Autodesk Fusion 360 part; units mm, degrees
sketch "Sketch1" plane through (0, 0, 0) normal (1, 0, 0) x (0, 0, -1)
  line L0 (0, 0) -> (-18.75, 0)
  line L1 (-18.75, 0) -> (-18.75, 20.75)
  line L2 (-18.75, 20.75) -> (0, 20.75)
  line L3 (0, 20.75) -> (0, 0)
  line L4 (-18.75, 20.75) -> (-18.75, 19)
  line L5 (-18.75, 0) -> (-18.75, 1.4)
  line L6 (-18.75, 19) -> (-22.75, 19)
  line L7 (-22.75, 19) -> (-22.75, 1.4)
  line L8 (-22.75, 1.4) -> (-18.75, 1.4)
  line L9 (-18.75, 1.4) -> (-18.75, 19)
  line L10 (-22.75, 19) -> (-22.75, 23.35)
  line L11 (-22.75, 1.4) -> (-22.75, -3.85)
  line L12 (-22.75, 23.35) -> (-60.15, 23.35)
  line L13 (-60.15, 23.35) -> (-60.15, -3.85)
  line L14 (-60.15, -3.85) -> (-22.75, -3.85)
  line L15 (-22.75, -3.85) -> (-22.75, 23.35)
  dimension "d1" = 18.75
  dimension "d2" = 20.75
  dimension "d4" = 1.75
  dimension "d6" = 4
  dimension "d7" = 4.35
  dimension "d9" = 37.4
sketch "Sketch3" plane through (0, 0, 0) normal (1, 0, 0) x (0, 0, -1)
  line L0 (-60.15, -3.85) -> (-60.15, 7.15)
  line L1 (-60.15, 7.15) -> (-39.15, 7.15)
  line L2 (-60.15, -3.85) -> (-22.75, -3.85)
  line L3 (-39.15, 7.15) -> (-39.15, -3.85)
  point P0 (-60.15, -3.85)
  dimension "d10" = 11
  dimension "d11" = 21
extrude "Extrude1" add sketch "Sketch3" along normal blind 6.15 makes body 1
sketch "Sketch4" plane through (6.15, 0, 0) normal (1, 0, 0) x (0, 0, -1)
  line L0 (-60.15, -3.85) -> (-39.15, -3.85)
  line L1 (-39.15, -3.85) -> (-39.15, 7.15)
  line L2 (-39.15, 7.15) -> (-60.15, 7.15)
  line L3 (-60.15, 7.15) -> (-60.15, -3.85)
  line L4 (-60.15, -3.85) -> (-18.75, -3.85)
  line L5 (-18.75, -3.85) -> (-18.75, 7.15)
  line L6 (-18.75, 7.15) -> (-60.15, 7.15)
  line L7 (-60.15, 7.15) -> (-60.15, -3.85)
  line L8 (-18.75, 1.4) -> (-18.75, 19)
extrude "Extrude2" add sketch "Sketch4" along normal blind 1.6 bodies 1
sketch "Sketch5" plane through (7.75, 0, 0) normal (1, 0, 0) x (0, 0, -1)
  line L0 (-18.75, -3.85) -> (-18.75, 7.15)
  line L1 (-18.75, 7.15) -> (-60.15, 7.15)
  line L2 (-60.15, 7.15) -> (-60.15, -3.85)
  line L3 (-60.15, -3.85) -> (-18.75, -3.85)
  line L4 (-60.15, -3.85) -> (0, -3.85)
  line L5 (0, -3.85) -> (0, 7.15)
  line L6 (0, 7.15) -> (-60.15, 7.15)
  line L7 (-60.15, 7.15) -> (-60.15, -3.85)
  line L8 (0, 20.75) -> (0, 0)
extrude "Extrude3" add sketch "Sketch5" along normal blind 7 bodies 1
sketch "Sketch6" plane through (0, 0, 60.15) normal (0, 0, 1) x (1, 0, 0)
  line L0 (0, 7.15) -> (0, -3.85)
  line L1 (0, -3.85) -> (14.75, -3.85)
  line L2 (14.75, -3.85) -> (14.75, 7.15)
  line L3 (14.75, 7.15) -> (0, 7.15)
  line L4 (0, -3.85) -> (-13.6, -3.85)
  dimension "d18" = 13.6
extrude "Extrude4" add sketch "Sketch3" along normal blind -14 and the other way blind 13.6 separate body makes body 2
extrude "Extrude5" add 1 faces at (-14, -0.1833, 46.15) along direction (-1, 0, 0) blind 6.15 on bodies 2 bodies 2
extrude "Extrude6" cut 1 faces at (-20.15, -0.1833, 46.15) along direction (1, 0, 0) blind 0.4 on bodies 2 bodies 2
sketch "Sketch7" plane through (-19.75, 0, 0) normal (-1, 0, 0) x (0, 0, 1)
  line L0 (39.15, -3.85) -> (60.15, -3.85)
  line L1 (60.15, -3.85) -> (60.15, 7.15)
  line L2 (60.15, 7.15) -> (39.15, 7.15)
  line L3 (39.15, 7.15) -> (39.15, -3.85)
  line L4 (60.15, 7.15) -> (18.75, 7.15)
  line L5 (18.75, 7.15) -> (18.75, -3.85)
  line L6 (18.75, -3.85) -> (60.15, -3.85)
  line L7 (60.15, -3.85) -> (60.15, 7.15)
  point P0 (18.75, -3.85)
extrude "Extrude7" add sketch "Sketch7" along normal blind 1.6 bodies 2
sketch "Sketch8" plane through (-21.35, 0, 0) normal (-1, 0, 0) x (0, 0, 1)
  line L0 (60.15, -3.85) -> (60.15, 7.15)
  line L1 (60.15, 7.15) -> (18.75, 7.15)
  line L2 (18.75, 7.15) -> (18.75, -3.85)
  line L3 (18.75, -3.85) -> (60.15, -3.85)
  line L4 (60.15, 7.15) -> (0, 7.15)
  line L5 (0, 7.15) -> (0, -3.85)
  line L6 (0, -3.85) -> (60.15, -3.85)
  line L7 (60.15, -3.85) -> (60.15, 7.15)
  point P0 (0, -3.85)
extrude "Extrude8" add sketch "Sketch8" along normal blind 7 bodies 2
sketch "Sketch9" plane through (0, 0, 0) normal (1, 0, 0) x (0, 0, -1)
  line L0 (-60.15, -3.85) -> (-25.95, -3.85)
  line L1 (-25.95, -3.85) -> (-22.75, 1.4)
  line L2 (-22.75, 1.4) -> (-18.75, 1.4)
  line L3 (-18.75, 1.4) -> (-18.75, 0)
  line L4 (-18.75, 0) -> (0, 0)
  line L5 (-25.95, -3.85) -> (0, -3.85)
  line L6 (0, -3.85) -> (0, 0)
  point P0 (-60.15, -3.85)
  point P1 (-22.75, 1.4)
  point P2 (-18.75, 1.4)
  point P3 (-18.75, 0)
  dimension "d31" = 34.2
extrude "Extrude9" add sketch "Sketch9" along normal blind 8 and the other way blind 24 bodies 1 2
sketch "Sketch10" plane through (0, -3.85, 0) normal (0, -1, 0) x (1, 0, 0)
  line L0 (-19.75, 25.95) -> (-19.75, 39.15)
  line L1 (-19.75, 39.15) -> (-13.6, 39.15)
  line L2 (-13.6, 39.15) -> (-13.6, 60.15)
  line L3 (-13.6, 60.15) -> (-28.35, 60.15)
  line L4 (-28.35, 60.15) -> (-28.35, 0)
  line L5 (-28.35, 0) -> (14.75, 0)
  line L6 (14.75, 0) -> (14.75, 60.15)
  line L7 (14.75, 60.15) -> (0, 60.15)
  line L8 (0, 60.15) -> (0, 39.15)
  line L9 (0, 39.15) -> (6.15, 39.15)
  line L10 (6.15, 39.15) -> (6.15, 25.95)
  line L11 (6.15, 25.95) -> (-19.75, 25.95)
  line L12 (-28.35, 60.15) -> (14.75, 60.15)
  line L13 (14.75, 60.15) -> (14.75, 0)
  line L14 (14.75, 0) -> (-28.35, 0)
  line L15 (-28.35, 0) -> (-28.35, 60.15)
extrude "Extrude10" add sketch "Sketch10" along normal blind 2 bodies 1
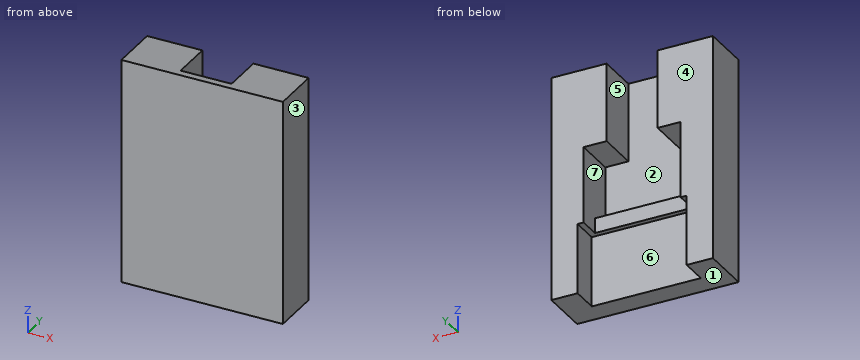
CAD build for the part. Positions are in the model's coordinates, mm. Face numbers are marked on the shaded views. A direction names the side the tool comes from. Round coordinates to 2 decimals unless told otherwise and drop trailing zeros. Write each loop counter-clockwise with the first axis right and the second up, starting at its lowest first coordinate (ties: lowest second). Pieces come first, ordered by that corner, then holes. Notation, with made-up numbers: (-9, -37) -> (9, -37) arc R23 ccw to (9, -10) -> close; hole circle Ø9 at (69, 46.5). An arc over 180 degrees is marked (long way). Answer as a JSON object with one key per item and string values.
(1) Band-saw the part on B-B, the plane x = -15.5. List the corners of the cut face in (y, z).
Reported:
{"outline": "(-5.85, 0) -> (0, 0) -> (0, 18.75) -> (1.4, 18.75) -> (1.4, 22.75) -> (-3.85, 25.95) -> (-3.85, 39.15) -> (7.15, 39.15) -> (7.15, 60.15) -> (-5.85, 60.15) -> close"}
(2) Band-saw the part on C-C, the plane z = 29. List the corners of the cut face in (x, y), then the cut area to 3 significant figures.
Reported:
{"outline": "(-28.35, -5.85) -> (14.75, -5.85) -> (14.75, 7.15) -> (6.15, 7.15) -> (6.15, -3.85) -> (-19.75, -3.85) -> (-19.75, 7.15) -> (-28.35, 7.15) -> close", "area": "275 mm^2"}
(3) Pin check, flat tips, straight feed: P1, Ø3.5, axis at x = -4, y = 3, coming from the -Z side; P2, Ø4.5, axis at x = -11.5, z = 20, coming from the +Y side; P3, Ø1.8, axis at x = 3.5, y = 4.5, coming from the -Z side; P4, Ø20.5, axis at x = -11.5, z = 51.5, coming from the +Y side. Stop position of each tip, or through.
Reported:
{"P1": "stops at z = 18.75", "P2": "stops at y = 1.4", "P3": "stops at z = 39.15", "P4": "stops at y = 7.15"}
(4) Probe probe 1 along X at (y, z) = (2, 10); probe 2 along X at (y, z) = (6.5, 34); probe 3 along Y at (x, z) = (-6, 22.5). List the from-to ranges inside material, lowest first. Write a range as [from, to].
Reported:
{"probe 1": "x = [-28.35, -21.35], [7.75, 14.75]", "probe 2": "x = [-28.35, -19.75], [6.15, 14.75]", "probe 3": "y = [-5.85, 1.4]"}
(5) Which spindle directions (+Z, -Z, +X, -X, +Y, -Y) get a long thin tool onto all of the face, cutting with end or side? Do the marked faces 4, 5, 6 and 7. Say none if no direction does.
Reported:
{"face 4": "+Z, -Z, +X, -X, +Y", "face 5": "+Z, +Y", "face 6": "-Z, +Y", "face 7": "+Y"}
(6) Band-saw the part on D-D, the plane z = 9.5. List the corners of the cut face in (x, y).
Reported:
{"outline": "(-28.35, -5.85) -> (14.75, -5.85) -> (14.75, 7.15) -> (7.75, 7.15) -> (7.75, 0) -> (-21.35, 0) -> (-21.35, 7.15) -> (-28.35, 7.15) -> close"}
(7) Two-plate mould, pull along Z, no slides. Class the marked faces 1, 2 and 3: +Z half, -Z half, draft (parallel to the pull), parting line (faces both ways), or undercut.
Reported:
{"face 1": "-Z half", "face 2": "undercut", "face 3": "draft"}
(8) Band-saw the part on A-A, the plane y = 3.25. List the corners of the cut face in (x, z), then the cut area to 3 significant figures.
Reported:
{"outline": "(-28.35, 0) -> (-21.35, 0) -> (-21.35, 18.75) -> (-19.75, 18.75) -> (-19.75, 39.15) -> (-13.6, 39.15) -> (-13.6, 60.15) -> (-28.35, 60.15) -> close; (0, 39.15) -> (6.15, 39.15) -> (6.15, 18.75) -> (7.75, 18.75) -> (7.75, 0) -> (14.75, 0) -> (14.75, 60.15) -> (0, 60.15) -> close", "area": "1,230 mm^2"}
